Geometry: final body of the model. Coordinates: model frame, mm. Give positions to 0.01 mm unless a question says otherwise; leave off trailing zeros. Write each loop counter-clockwise with the first axis right and the second up, starting at its lowest first coordinate (ties: lowest second). Pieces come first, ordered by that corner, then holes. Notation, with made-up numbers: (79, -30) -> (109, -30) arc R6 cw to (109, -21) -> close; hole circle Ø3 at (20.5, 52). An arc over 180 degrees is marked (long way). Use CSV: the item, a comma, the result in double quotes. Start each with the question number.
1) Section A-A (x = 29.5). Output: boundary loops of the cut face in (y, z), plus the area to 3 significant figures.
2) Material intervals for line 1 (Z direction, x = 3, y = -2.25); line 2 (X direction, y = -2, z = -26); line 3 (Y direction, x = -12, z = 3), sorted ascending. Write a range as [from, to].
3) Section C-C (z = -86.5). Output: boundary loops of the cut face in (x, y).
4) Section B-B (x = 12). Output: boundary loops of the cut face in (y, z).
5) Contact query for a flat-ended pin moving along its axis: P1, Ø3, axis at x = 24, y = 0, coming from the +Z side. Output: stop coordinate, or through.
```python
from build123d import *

# Parameters (mm, degrees)
SKETCH_1_W      = 104
SKETCH_1_H      = 9
SKETCH_1_R      = 2.5
EXTRUDE_1_DEPTH = 5
SKETCH_2_W      = 3
SKETCH_2_H      = 9
EXTRUDE_2_DEPTH = 90


with BuildPart() as part:
    # 草圖1 → 填料-伸長1 (new body)
    with BuildSketch(Plane.XY):
        Rectangle(SKETCH_1_W, SKETCH_1_H)
        with Locations((-36, 0)):
            Circle(SKETCH_1_R, mode=Mode.SUBTRACT)
        with Locations((-24, 0)):
            Circle(SKETCH_1_R, mode=Mode.SUBTRACT)
        with Locations((-12, 0)):
            Circle(SKETCH_1_R, mode=Mode.SUBTRACT)
        Circle(SKETCH_1_R, mode=Mode.SUBTRACT)
        with Locations((12, 0)):
            Circle(SKETCH_1_R, mode=Mode.SUBTRACT)
        with Locations((24, 0)):
            Circle(SKETCH_1_R, mode=Mode.SUBTRACT)
        with Locations((36, 0)):
            Circle(SKETCH_1_R, mode=Mode.SUBTRACT)
    extrude_1 = extrude(amount=EXTRUDE_1_DEPTH)

    # 草圖2 → 填料-伸長2 (add)
    with BuildSketch(Plane(origin=(0, 0, 0), x_dir=(-1, 0, 0), z_dir=(0, 0, -1))):
        with Locations((-50.5, 0)):
            Rectangle(SKETCH_2_W, SKETCH_2_H)
        with Locations((50.5, 0)):
            Rectangle(SKETCH_2_W, SKETCH_2_H)
    extrude_2 = extrude(amount=EXTRUDE_2_DEPTH)

    # 鏡射4: 填料-伸長1, 填料-伸長2 across plane
    add(extrude_1.mirror(Plane(origin=(0, 0, -90), x_dir=(1, 0, 0), z_dir=(0, 0, -1))))
    add(extrude_2.mirror(Plane(origin=(0, 0, -90), x_dir=(1, 0, 0), z_dir=(0, 0, -1))))


solid = part.part
```
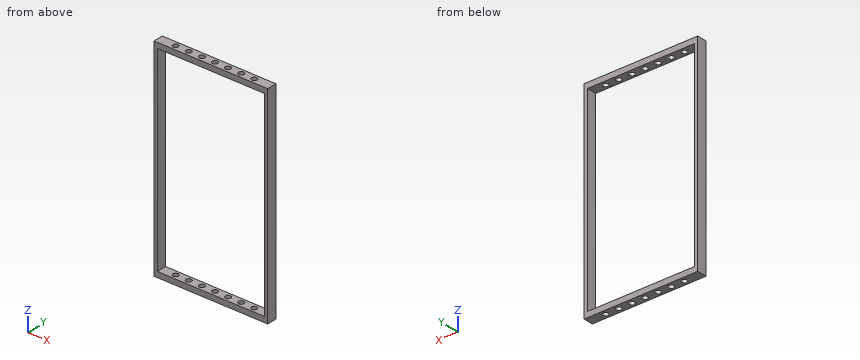
Answers follow:
1,outline,"(-4.5, -185) -> (4.5, -185) -> (4.5, -180) -> (-4.5, -180) -> close; (-4.5, 0) -> (4.5, 0) -> (4.5, 5) -> (-4.5, 5) -> close"
1,area,"90.0 mm^2"
2,line 1,"z = [-185, -180], [0, 5]"
2,line 2,"x = [-52, -49], [49, 52]"
2,line 3,"y = [-4.5, -2.5], [2.5, 4.5]"
3,outline,"(-52, -4.5) -> (-49, -4.5) -> (-49, 4.5) -> (-52, 4.5) -> close; (49, -4.5) -> (52, -4.5) -> (52, 4.5) -> (49, 4.5) -> close"
4,outline,"(-4.5, -185) -> (-2.5, -185) -> (-2.5, -180) -> (-4.5, -180) -> close; (-4.5, 0) -> (-2.5, 0) -> (-2.5, 5) -> (-4.5, 5) -> close; (2.5, -185) -> (4.5, -185) -> (4.5, -180) -> (2.5, -180) -> close; (2.5, 0) -> (4.5, 0) -> (4.5, 5) -> (2.5, 5) -> close"
5,P1,"passes through"
